The listing builds one solid part. Answer for the finished solid, in the listing's coordinates (mm). A direction names the side the tool comes from. Give positions to 0.01 mm unless a question says otherwise; leave off trailing zeros. Order: outer loops, then holes, each group sorted by start corner. A loop starts at its lowest first (then second) coordinate and runs counter-clockwise, first axis right, second up. Notation, with made-up numbers: (-5, -32) - (18, -32) arc R17 ccw to (18, -12) - close; hole circle Ø7 at (59, 12). An arc over 180 degrees is marked (long way). Answer as a JSON object with one key per item and string values. Group by question number.
Q1. The mould has two halves that part along X. Classify faces 1 (the face through (18, 0, 2)), 2 (the face through (31.75, 3, 5)), 3 (the face through (35.56, 3, 5)): released by +X, released by -X, zero draft, split by the parting line, or undercut.
Q2. A cutting plane is placed at B-B, the plane y = 5.5. Give the vertices of the cut face in (x, z), and give its area (3 significant figures).
Q3. Consider line 1 (X direction, y = 1, z = 6.25); line 2 (Z direction, x = 16, y = 3.25); line 3 (X direction, y = 1, z = 1.25). Determine where each line is inside the solid, lowest interval first.
Q4. A cutting plane is placed at C-C, the plane x = 15. Give the vertices of the cut face in (y, z), and give its area (3 significant figures).
Q5. For faces 4 (the face through (34, 3, 7.62)), 5 (the face through (3.81, 3, 5)), determine the directions among +Z, -Z, +X, -X, +Y, -Y from which every point of the face is accessible in a straight line to the end or side of a thin tool.
Q6. A cutting plane is placed at A-A, the plane z = 5.75. Give the vertices of the cut face in (x, y).
from build123d import *

# Parameters (mm, degrees)
SKETCH1_W           = 35.56
SKETCH1_H           = 7.62
BOSS_EXTRUDE1_DEPTH = 6.35
SKETCH2_W           = 27.94
SKETCH2_H           = 5.08
CUT_EXTRUDE1_DEPTH  = 37.917482309
FILLET1_R           = 2.54


with BuildPart() as part:
    # Sketch1 → Boss-Extrude1 (new body)
    with BuildSketch(Plane(origin=(0, 0, 0), x_dir=(1, 0, 0), z_dir=(0, 1, 0))):
        with Locations((17.78, -3.81)):
            Rectangle(SKETCH1_W, SKETCH1_H)
    extrude(amount=BOSS_EXTRUDE1_DEPTH)

    # Sketch2 → Cut-Extrude1 (cut, through all)
    with BuildSketch(Plane(origin=(0, 6.35, 0), x_dir=(1, 0, 0), z_dir=(0, 1, 0))):
        with Locations((17.78, -5.08)):
            Rectangle(SKETCH2_W, SKETCH2_H)
    extrude(amount=-CUT_EXTRUDE1_DEPTH, mode=Mode.SUBTRACT)

    # Fillet1
    fillet1_edges = [part.edges().sort_by_distance(p)[0] for p in [
        (0, 3.175, 0),
        (35.56, 3.175, 0),
    ]]
    fillet(fillet1_edges, radius=FILLET1_R)


solid = part.part
Reply:
{
 "1": {"face 1": "zero draft", "face 2": "undercut", "face 3": "released by +X"},
 "2": {"outline": "(0, 2.54) arc R2.54 ccw to (2.54, 0) - (33.02, 0) arc R2.54 ccw to (35.56, 2.54) - (35.56, 7.62) - (31.75, 7.62) - (31.75, 2.54) - (3.81, 2.54) - (3.81, 7.62) - (0, 7.62) - close", "area": "126 mm^2"},
 "3": {"line 1": "x = 0 to 3.81, 31.75 to 35.56", "line 2": "z = 0 to 2.54", "line 3": "x = 0.35 to 35.21"},
 "4": {"outline": "(0, 0) - (6.35, 0) - (6.35, 2.54) - (0, 2.54) - close", "area": "16.1 mm^2"},
 "5": {"face 4": "+Z, +X, -X, +Y, -Y", "face 5": "+Z, +Y, -Y"},
 "6": {"outline": "(0, 0) - (3.81, 0) - (3.81, 6.35) - (0, 6.35) - close; (31.75, 0) - (35.56, 0) - (35.56, 6.35) - (31.75, 6.35) - close"}
}
